from build123d import *

# Parameters (mm, degrees)
BOX039_W               = 7.4
BOX039_H               = 1
BOX039_DEPTH           = 3.95
BOX038_W               = 6.7
BOX038_H               = 2
BOX038_DEPTH           = 0.45
CYLINDER008_R          = 0.45
CYLINDER008_DEPTH      = 0.4
CYLINDER_R             = 0.45
CYLINDER_DEPTH         = 0.4
BOX028_W               = 7.4
BOX028_H               = 7
BOX028_DEPTH           = 3.85
BOX037_W               = 0.25
BOX037_H               = 2.2
BOX037_DEPTH           = 0.5
BOX036_W               = 0.25
BOX036_H               = 2.2
BOX036_DEPTH           = 0.5
BOX035_W               = 0.25
BOX035_H               = 2.2
BOX035_DEPTH           = 0.5
BOX034_W               = 0.25
BOX034_H               = 2.2
BOX034_DEPTH           = 0.5
BOX033_W               = 0.25
BOX033_H               = 2.2
BOX033_DEPTH           = 0.5
BOX032_W               = 2
BOX032_H               = 3
BOX032_DEPTH           = 2
BOX032_PLACEMENT_ANGLE = 45
BOX031_W               = 2
BOX031_H               = 3
BOX031_DEPTH           = 2
BOX031_PLACEMENT_ANGLE = 45
BOX029_W               = 5.7
BOX029_H               = 1
BOX029_DEPTH           = 2
BOX029_PLACEMENT_ANGLE = 15
BOX030_W               = 5.7
BOX030_H               = 1
BOX030_DEPTH           = 2


with BuildPart() as cube031:
    # Box039 → Box039 (new body)
    with BuildSketch(Plane(origin=(0.15, 8.6, -0.1), x_dir=(1, 0, 0), z_dir=(0, 0, 1))):
        with Locations((3.7, 0.5)):
            Rectangle(BOX039_W, BOX039_H)
    extrude(amount=BOX039_DEPTH)


with BuildPart() as cube030:
    # Box038 → Box038 (new body)
    with BuildSketch(Plane(origin=(0.5, 7.7, -0.1), x_dir=(1, 0, 0), z_dir=(0, 0, 1))):
        with Locations((3.35, 1)):
            Rectangle(BOX038_W, BOX038_H)
    extrude(amount=BOX038_DEPTH)


with BuildPart() as cone001:
    # Cone001 → Cone001 (revolve)
    with BuildSketch(Plane(origin=(6.05, 5.9, -0.8), x_dir=(1, 0, 0), z_dir=(0, -1, 0))):
        Polygon((0, 0), (0.25, 0), (0.45, 0.4), (0, 0.4), align=None)
    revolve(axis=Axis((6.05, 5.9, -0.8), (0, 0, 1)))


with BuildPart() as fusion002:
    # Cylinder008 → Cylinder008 (new body)
    with BuildSketch(Plane(origin=(6.05, 5.9, -0.4), x_dir=(1, 0, 0), z_dir=(0, 0, 1))):
        Circle(CYLINDER008_R)
    extrude(amount=CYLINDER008_DEPTH)

    # Fusion002: union Cone001
    add(cone001.part)


with BuildPart() as cone:
    # Cone → Cone (revolve)
    with BuildSketch(Plane(origin=(1.65, 5.9, -0.8), x_dir=(1, 0, 0), z_dir=(0, -1, 0))):
        Polygon((0, 0), (0.25, 0), (0.45, 0.4), (0, 0.4), align=None)
    revolve(axis=Axis((1.65, 5.9, -0.8), (0, 0, 1)))


with BuildPart() as fusion:
    # Cylinder → Cylinder (new body)
    with BuildSketch(Plane(origin=(1.65, 5.9, -0.4), x_dir=(1, 0, 0), z_dir=(0, 0, 1))):
        Circle(CYLINDER_R)
    extrude(amount=CYLINDER_DEPTH)

    # Fusion: union Cone
    add(cone.part)


with BuildPart() as fusion004:
    # Box028 → Box028 (new body)
    with BuildSketch(Plane(origin=(0.15, 2.2, 0), x_dir=(1, 0, 0), z_dir=(0, 0, 1))):
        with Locations((3.7, 3.5)):
            Rectangle(BOX028_W, BOX028_H)
    extrude(amount=BOX028_DEPTH)

    # Fusion003: union Fusion
    add(fusion.part)

    # Fusion004: union Fusion002
    add(fusion002.part)


with BuildPart() as cube029:
    # Box037 → Box037 (new body)
    with BuildSketch(Plane(origin=(5.5, 0.1, 1.65), x_dir=(1, 0, 0), z_dir=(0, 0, 1))):
        with Locations((0.125, 1.1)):
            Rectangle(BOX037_W, BOX037_H)
    extrude(amount=BOX037_DEPTH)


with BuildPart() as cube028:
    # Box036 → Box036 (new body)
    with BuildSketch(Plane(origin=(4.6, 0.1, 1.65), x_dir=(1, 0, 0), z_dir=(0, 0, 1))):
        with Locations((0.125, 1.1)):
            Rectangle(BOX036_W, BOX036_H)
    extrude(amount=BOX036_DEPTH)


with BuildPart() as cube027:
    # Box035 → Box035 (new body)
    with BuildSketch(Plane(origin=(3.7, 0.1, 1.65), x_dir=(1, 0, 0), z_dir=(0, 0, 1))):
        with Locations((0.125, 1.1)):
            Rectangle(BOX035_W, BOX035_H)
    extrude(amount=BOX035_DEPTH)


with BuildPart() as cube026:
    # Box034 → Box034 (new body)
    with BuildSketch(Plane(origin=(2.8, 0.1, 1.65), x_dir=(1, 0, 0), z_dir=(0, 0, 1))):
        with Locations((0.125, 1.1)):
            Rectangle(BOX034_W, BOX034_H)
    extrude(amount=BOX034_DEPTH)


with BuildPart() as cube025:
    # Box033 → Box033 (new body)
    with BuildSketch(Plane(origin=(1.9, 0.1, 1.65), x_dir=(1, 0, 0), z_dir=(0, 0, 1))):
        with Locations((0.125, 1.1)):
            Rectangle(BOX033_W, BOX033_H)
    extrude(amount=BOX033_DEPTH)


with BuildPart() as cube024:
    # Box032 → Box032 (new body)
    with BuildSketch(Plane.XY):
        with Locations((1, 1.5)):
            Rectangle(BOX032_W, BOX032_H)
    extrude(amount=BOX032_DEPTH)


with BuildPart() as cube024_1:
    # Box032 placement: moved
    add(cube024.part.moved(Location((6.8, 0, -1.4))).rotate(Axis((6.8, 0, -1.4), (0, -1, 0)), BOX032_PLACEMENT_ANGLE))


with BuildPart() as cube023:
    # Box031 → Box031 (new body)
    with BuildSketch(Plane.XY):
        with Locations((1, 1.5)):
            Rectangle(BOX031_W, BOX031_H)
    extrude(amount=BOX031_DEPTH)


with BuildPart() as cube023_1:
    # Box031 placement: moved
    add(cube023.part.moved(Location((-0.5, 0, 0))).rotate(Axis((-0.5, 0, 0), (0, 1, 0)), BOX031_PLACEMENT_ANGLE))


with BuildPart() as cube021:
    # Box029 → Box029 (new body)
    with BuildSketch(Plane.XY):
        with Locations((2.85, 0.5)):
            Rectangle(BOX029_W, BOX029_H)
    extrude(amount=BOX029_DEPTH)


with BuildPart() as cube021_1:
    # Box029 placement: moved
    add(cube021.part.moved(Location((1, 0.65, 0.2))).rotate(Axis((1, 0.65, 0.2), (1, 0, 0)), BOX029_PLACEMENT_ANGLE))


with BuildPart() as plastic_guts:
    # Box030 → Box030 (new body)
    with BuildSketch(Plane(origin=(1, 1.2, 0.5), x_dir=(1, 0, 0), z_dir=(0, 0, 1))):
        with Locations((2.85, 0.5)):
            Rectangle(BOX030_W, BOX030_H)
    extrude(amount=BOX030_DEPTH)

    # Cut026: cut Cube021
    add(cube021_1.part, mode=Mode.SUBTRACT)

    # Cut027: cut Cube023
    add(cube023_1.part, mode=Mode.SUBTRACT)

    # Cut028: cut Cube024
    add(cube024_1.part, mode=Mode.SUBTRACT)

    # Cut029: cut Cube025
    add(cube025.part, mode=Mode.SUBTRACT)

    # Cut030: cut Cube026
    add(cube026.part, mode=Mode.SUBTRACT)

    # Cut031: cut Cube027
    add(cube027.part, mode=Mode.SUBTRACT)

    # Cut032: cut Cube028
    add(cube028.part, mode=Mode.SUBTRACT)

    # Cut033: cut Cube029
    add(cube029.part, mode=Mode.SUBTRACT)

    # Fusion005: union Fusion004
    add(fusion004.part)

    # Cut034: cut Cube030
    add(cube030.part, mode=Mode.SUBTRACT)

    # Cut035: cut Cube031
    add(cube031.part, mode=Mode.SUBTRACT)


solid = plastic_guts.part
The listing builds one solid part. Answer for the finished solid, in the listing's coordinates (mm). A direction names the side the tool comes from. Give positions to 0.01 mm unless a question says otherwise; leave off trailing zeros. Loops run counter-clockwise (first coordinate to the right, second up) from the corner with the lowest first, then second, coordinate; pieces in that order, holes last. Notation, with made-up numbers: (52.5, 85.5) - (70.5, 85.5) arc R22 cw to (70.5, 110.5) - close; hole circle Ø2 at (29, 22.5). An arc over 180 degrees is marked (long way). Answer as a JSON object with one key per item and string values.
1. For a pull along X with two mould halves and no side action, classify faces 1 (the flat face through (4, 2, 2.5)), 2 (the flat face through (1, 2, 2)), 3 (the flat face through (4, 8, 0.35)) as pulls with the +X half, pulls with the -X half, needs draft (parallel to the pull), parting line crosses it, or undercut.
Determined:
{"face 1": "needs draft", "face 2": "pulls with the -X half", "face 3": "undercut"}
2. Find the intervals of material crossed by L1, parallel to Z at x = 3.25, y = 4; L2, parallel to Y at x = 2.75, z = 2.95; L3, parallel to Y at x = 1, z = 0.1, in increasing order. Write a range as [from, to].
Determined:
{"L1": "[0, 3.85]", "L2": "[2.2, 8.6]", "L3": "[2.2, 7.7]"}
3. A cutting plane is placed at C-C (z = 2.4). Write down the section's boundary in (x, y).
Determined:
{"outline": "(0.15, 2.2) - (1, 2.2) - (1, 1.2) - (6.7, 1.2) - (6.7, 2.2) - (7.55, 2.2) - (7.55, 8.6) - (0.15, 8.6) - close"}
4. A cutting plane is placed at A-A (y = 8). Write down the section's boundary in (x, z).
Determined:
{"outline": "(0.15, 0) - (0.5, 0) - (0.5, 0.35) - (7.2, 0.35) - (7.2, 0) - (7.55, 0) - (7.55, 3.85) - (0.15, 3.85) - close"}
5. A cutting plane is placed at B-B (x = 2.5). Write down the section's boundary in (y, z).
Determined:
{"outline": "(1.2, 2.01) - (1.6, 0.5) - (2.2, 0.5) - (2.2, 0) - (7.7, 0) - (7.7, 0.35) - (8.6, 0.35) - (8.6, 3.85) - (2.2, 3.85) - (2.2, 2.5) - (1.2, 2.5) - close"}
6. A cutting plane is placed at D-D (y = 5.9). Write down the section's boundary in (x, z).
Determined:
{"outline": "(0.15, 0) - (1.2, 0) - (1.2, -0.4) - (1.4, -0.8) - (1.9, -0.8) - (2.1, -0.4) - (2.1, 0) - (5.6, 0) - (5.6, -0.4) - (5.8, -0.8) - (6.3, -0.8) - (6.5, -0.4) - (6.5, 0) - (7.55, 0) - (7.55, 3.85) - (0.15, 3.85) - close"}
7. For faces 4 (the flat face through (6.7, 2, 2)), 5 (the cylindrical face through (6.26, 5.5, -0.2)), 6 (the flat face through (6.28, 1.89, 0.91)), 7 (the flat face through (1.41, 1.89, 0.92)), determine the directions among +Z, -Z, +X, -X, +Y, -Y from which every point of the face is accessible in a straight line to the end or side of a thin tool.
Determined:
{"face 4": "+Z, -Z, +X, -Y", "face 5": "-Z", "face 6": "-Z, +X, -Y", "face 7": "-Z, -X, -Y"}
